Drawing for the job (mm, zero at the part's lowest x, y, z). A direction names the side the tool comes from. Give positions to 0.01 mm unless a question says otherwise; leave off trailing zeros. Order: outer loops, then holes, each group sorted by start corner. A loop starts at its lowest first (then second) coordinate and runs counter-clockwise, first axis right, second up. Notation, with made-up numbers: (-39.5, -15.75) -> (-13.5, -15.75) arc R5 ccw to (-13.5, -8.75) -> close; hole circle Ø7 at (38, 55.25). An arc over 180 degrees is marked (long way). One line per item, written item: value. Start each with the question number.
(1) Saw through at C-C on x = 27. Give the cut face in (y, z).
(2) Pin check, flat tips, straight feed: pin 1 (3 mm diameter, centred on y = 10.5, z = 36.5, fed in from +X); pin 2 (4 mm diameter, centred on x = 48, z = 8, fed in from +Y); pin 3 (2 mm diameter, centred on x = 64, z = 32.5, fed in from -Y). Stop position of each tip, or through.
(3) Two-plate mould, pull along X, no slides. Class the marked faces 4 and 5: +X half, -X half, draft (parallel to the pull), parting line (faces both ways), or undercut.
(4) Saw through at B-B on z = 6. Give the cut face in (x, y).
(5) Which spindle directions (+Z, -Z, +X, -X, +Y, -Y) get a long thin tool onto all of the face, cutting with end or side? Do the marked faces 1, 2 and 3. Say none if no direction does.
(6) Probe line 1 (Z direction, x = 61, y = 9); line 2 (X direction, y = 14.75, z = 16.5) (1 decimal); line 3 (X direction, y = 18.75, z = 2) (1 decimal). List the from-to ranges inside material, lowest first.
(7) Saw through at A-A on z = 12. Give the cut face in (x, y).
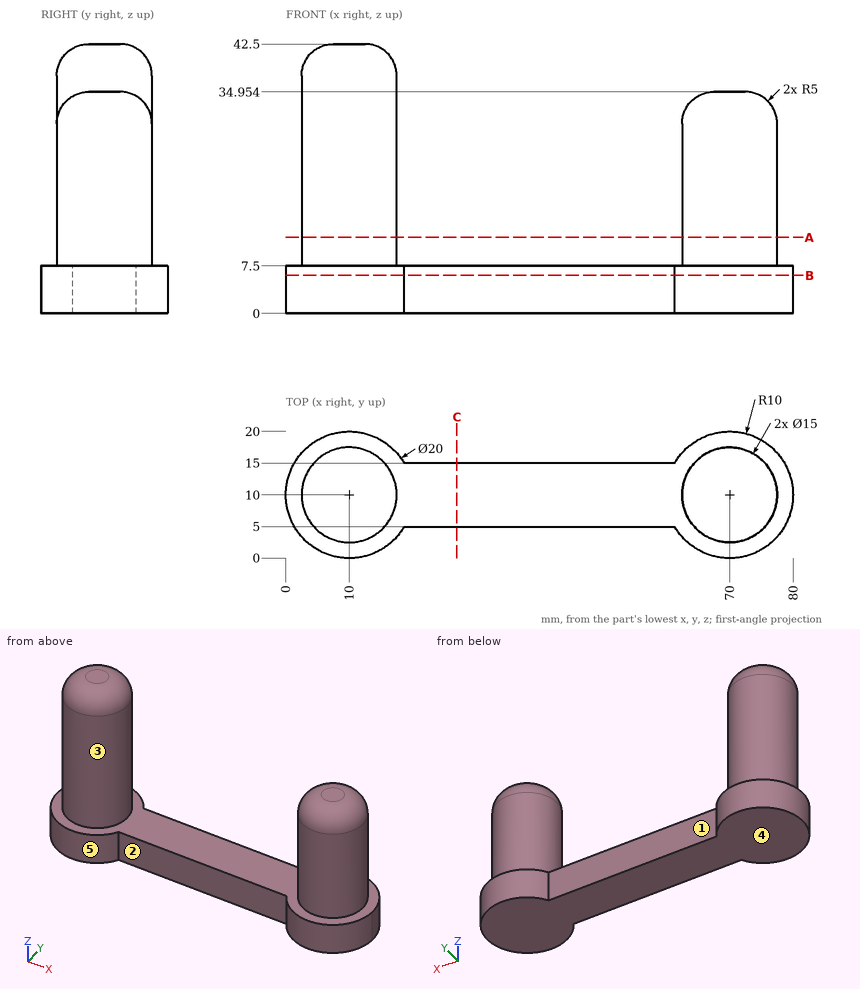
Results below:
1. outline: (5, 0) -> (15, 0) -> (15, 7.5) -> (5, 7.5) -> close
2. pin 1: stops at x = 17.5
2. pin 2: stops at y = 15
2. pin 3: stops at y = 5.15
3. face 4: draft
3. face 5: undercut
4. outline: (18.66, 5) -> (61.34, 5) arc R10 ccw (long way) to (61.34, 15) -> (18.66, 15) arc R10 ccw (long way) to start
5. face 1: +Z, -Z, +Y
5. face 2: +Z, -Z, -Y
5. face 3: +Z
6. line 1: z = 0 to 7.5
6. line 2: x = 4.2 to 15.8, 64.2 to 75.8
6. line 3: x = 5.2 to 14.8, 65.2 to 74.8
7. outline: circle Ø15 at (10, 10); circle Ø15 at (70, 10)
